```python
from build123d import *

# Parameters (mm, degrees)
SKETCH1_W           = 42
SKETCH1_H           = 42
SKETCH1_W_2         = 36
SKETCH1_H_2         = 36
BOSS_EXTRUDE1_DEPTH = 24
SKETCH3_R           = 11
CUT_EXTRUDE1_DEPTH  = 1
SKETCH5_R           = 9
CUT_EXTRUDE2_DEPTH  = 4
SKETCH14_W          = 42
SKETCH14_H          = 42
BOSS_EXTRUDE3_DEPTH = 1
CIRPATTERN1_COUNT   = 4
FILLET1_R           = 2
SKETCH15_W          = 22
SKETCH15_H          = 22
CUT_EXTRUDE3_DEPTH  = 26


with BuildPart() as part:
    # Sketch1 → Boss-Extrude1 (new body)
    with BuildSketch(Plane.XY):
        Rectangle(SKETCH1_W, SKETCH1_H)
        Rectangle(SKETCH1_W_2, SKETCH1_H_2, mode=Mode.SUBTRACT)
    extrude(amount=BOSS_EXTRUDE1_DEPTH)

    # Sketch3 → Cut-Extrude1 (cut)
    with BuildSketch(Plane.ZY.offset(-18)):
        Circle(SKETCH3_R)
    cut_extrude1 = extrude(amount=-CUT_EXTRUDE1_DEPTH, mode=Mode.SUBTRACT)

    # Sketch5 → Cut-Extrude2 (cut, through all)
    with BuildSketch(Plane.ZY.offset(-18)):
        Circle(SKETCH5_R)
    cut_extrude2 = extrude(amount=-CUT_EXTRUDE2_DEPTH, mode=Mode.SUBTRACT)

    # Sketch14 → Boss-Extrude3 (add)
    with BuildSketch(Plane.XY.offset(24)):
        Rectangle(SKETCH14_W, SKETCH14_H)
    extrude(amount=BOSS_EXTRUDE3_DEPTH)

    # CirPattern1: Cut-Extrude1, Cut-Extrude2 ×4 about axis
    cirpattern1_axis = Axis((0, 0, 0), (0, 0, 1))
    for i in range(1, CIRPATTERN1_COUNT):
        add(cut_extrude1.rotate(cirpattern1_axis, i * 360 / CIRPATTERN1_COUNT), mode=Mode.SUBTRACT)
        add(cut_extrude2.rotate(cirpattern1_axis, i * 360 / CIRPATTERN1_COUNT), mode=Mode.SUBTRACT)

    # Fillet1
    fillet1_edges = [part.edges().sort_by_distance(p)[0] for p in [
        (21, -21, 12.5),
        (-21, -21, 12.5),
        (-21, 21, 12.5),
        (21, 21, 12.5),
    ]]
    fillet(fillet1_edges, radius=FILLET1_R)

    # Sketch15 → Cut-Extrude3 (cut, through all)
    with BuildSketch(Plane.XY.offset(25)):
        Rectangle(SKETCH15_W, SKETCH15_H)
    extrude(amount=-CUT_EXTRUDE3_DEPTH, mode=Mode.SUBTRACT)


solid = part.part
```
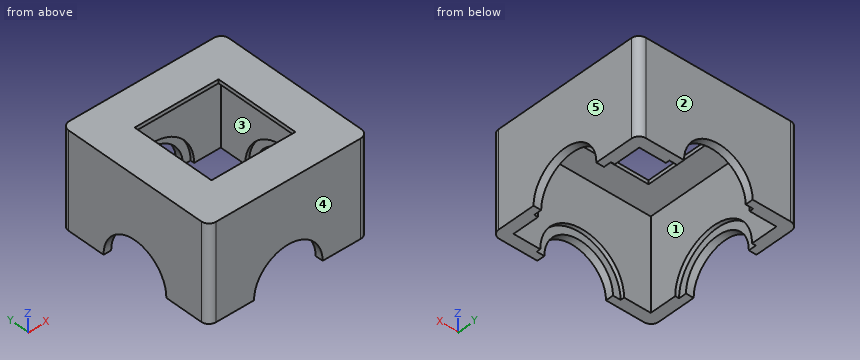
Geometry: final body of the model. Coordinates: model frame, mm. Face numbers are marked on the shaded views. A direction names the side the tool comes from. Coordinates: 2 decimals unless noted, no trailing zeros. Order: outer loops, then holes, each group sorted by start corner. A loop starts at its lowest first (then second) coordinate and runs counter-clockwise, first axis right, second up. Notation, with made-up numbers: (18.5, -9) -> (30.5, -9) arc R16 cw to (30.5, 16) -> close; hole circle Ø11 at (58.5, -32). An arc over 180 degrees is marked (long way). Write each question's results on one line, items separated by ' | '. Start each with the question number.
1) Set-up query: the marked faces 1 and 2. Return all of +Z, -Z, +X, -X, +Y, -Y with unobstructed straight access to the full face (end or side cutting, diameter ignored); none if empty.
2) Material intervals for line 1 along X through (y, z) = (15, 22.25); line 2 along X through (y, z) = (-7, 6.5), sorted ascending.
3) Cut plane C-C, the plane z = 23. Output: boundary loops of the cut face in (x, y), and give its area (3 significant figures).
4) Cut plane A-A, the plane x = 0. Output: boundary loops of the cut face in (y, z), and give its area (3 significant figures).
5) Cut plane D-D, the plane x = 15. Output: boundary loops of the cut face in (y, z), and give its area (3 significant figures).
6) Mould query, pull axis Y, two halves, no side actions, for the marked faces 3, 4 and 5. Classes: released by +Y, released by -Y, zero draft, split by the parting line, or undercut.
7) First-contact query: pin 1 (11 mm diameter, centred on x = -7, y = 0.5, fed in from -Z). Flat tip, straight axial feed; report the tip coordinate or a pass-through.
Checks:
1) face 1: -Z | face 2: +Z, -Z, +X, -X, +Y
2) line 1: -21 to -18, 18 to 21 | line 2: -21 to -19, 19 to 21
3) outline: (-21, -19) arc R2 ccw to (-19, -21) -> (19, -21) arc R2 ccw to (21, -19) -> (21, 19) arc R2 ccw to (19, 21) -> (-19, 21) arc R2 ccw to (-21, 19) -> close; hole (-18, -18) -> (18, -18) -> (18, 18) -> (-18, 18) -> close | area: 465 mm^2
4) outline: (-21, 9) -> (-19, 9) -> (-19, 11) -> (-18, 11) -> (-18, 24) -> (-11, 24) -> (-11, 25) -> (-21, 25) -> close; (11, 24) -> (18, 24) -> (18, 11) -> (19, 11) -> (19, 9) -> (21, 9) -> (21, 25) -> (11, 25) -> close | area: 106 mm^2
5) outline: (-21, 0) -> (-18, 0) -> (-18, 24) -> (18, 24) -> (18, 0) -> (21, 0) -> (21, 25) -> (-21, 25) -> close | area: 186 mm^2
6) face 3: undercut | face 4: released by -Y | face 5: zero draft
7) pin 1: z = 24
